Build history of the part. All positions in model axes, mm. A direction names the side the tool comes from. Round coordinates to 2 decimals unless told otherwise and drop trailing zeros. Write each loop counter-clockwise with the first axis right and the second up, starting at its lowest first coordinate (ties: lowest second). Pieces come first, ordered by that corner, then holes.
from build123d import *

# Parameters (mm, degrees)
SKETCH1_W                = 39
SKETCH1_H                = 70
BASE_DEPTH               = 4.5
SKETCH2_W                = 4
SKETCH2_H                = 62
WALLS_DEPTH              = 7.5
SKETCH3_W                = 10
SKETCH3_H                = 7.5
PWR_CONNECTOR_HOLE_DEPTH = 4
SKETCH4_W                = 7.5
SKETCH4_H                = 8
GPS_CONNECTOR_HOLE_DEPTH = 4
SKETCH5_R                = 1.25
MOUNTING_HOLES_DEPTH     = 4
GPS_MOUNT_DEPTH          = 4
SKETCH11_W               = 17
SKETCH11_H               = 1
SKETCH11_W_2             = 12
SKETCH11_H_2             = 3
PWR_CABLE_HOLDER1_DEPTH  = 4
PWR_FILLET2_R            = 1
PWR_FILLET3_R            = 0.5
SKETCH15_R               = 6
BALLON_MOUNT_DEPTH       = 70
SKETCH16_R               = 2.25
BALLOON_MOUNT_HOLE_DEPTH = 70
SKETCH21_R               = 2.25
SAFETY_MOUNT_DEPTH       = 4.5
SKETCH22_W               = 35
SKETCH22_H               = 66
LID_HOLE_DEPTH           = 7.5
SKETCH25_W               = 3.5
SKETCH25_H               = 66
CORRECTION_DEPTH         = 2
FILLET4_R                = 0.75
FILLET5_R                = 1
SKETCH12_W               = 7
SKETCH12_H               = 2.5
SKETCH12_W_2             = 2
SKETCH12_H_2             = 2
CUT_EXTRUDE2_DEPTH       = 1.99
SKETCH13_W               = 2.326586719
SKETCH13_H               = 10
CUT_EXTRUDE3_DEPTH       = 2
FILLET6_R                = 1
FILLET7_R                = 1
FILLET8_START            = 4
FILLET8_DEPTH            = 12.5
FILLET8_START_2          = 9.5
FILLET8_2_DEPTH          = 7


with BuildPart() as part:
    # Sketch1 → Base (new body)
    with BuildSketch(Plane.XY):
        with Locations((19.5, 35)):
            Rectangle(SKETCH1_W, SKETCH1_H)
    extrude(amount=BASE_DEPTH)

    # Sketch2 → Walls (add)
    with BuildSketch(Plane.XY.offset(4.5)):
        Polygon((39, 66), (39, 70), (0, 70), (0, 66), (4, 66), (35, 66), align=None)
        with Locations((37, 35)):
            Rectangle(SKETCH2_W, SKETCH2_H)
        Polygon((4, 66), (0, 66), (0, 0), (4, 0), (4, 4), align=None)
        Polygon((39, 0), (39, 4), (35, 4), (4, 4), (4, 0), align=None)
    extrude(amount=WALLS_DEPTH)

    # Sketch3 → PWR connector hole (cut)
    with BuildSketch(Plane(origin=(0, 4, 0), x_dir=(1, 0, 0), z_dir=(0, 1, 0))):
        with Locations((14.5, -8.25)):
            Rectangle(SKETCH3_W, SKETCH3_H)
    extrude(amount=-PWR_CONNECTOR_HOLE_DEPTH, mode=Mode.SUBTRACT)

    # Sketch4 → GPS connector hole (cut)
    with BuildSketch(Plane.ZY.offset(-35)):
        with Locations((8.25, 18.5)):
            Rectangle(SKETCH4_W, SKETCH4_H)
    extrude(amount=-GPS_CONNECTOR_HOLE_DEPTH, mode=Mode.SUBTRACT)

    # Sketch5 → Mounting holes (cut)
    with BuildSketch(Plane.XY.offset(4.5)):
        with Locations((7.25, 7.25)):
            Circle(SKETCH5_R)
        with Locations(Location((31.75, 7.25, 0), (0, 0, 180))):
            Circle(SKETCH5_R)
        with Locations(Location((7.25, 62.75, 0), (0, 0, 180))):
            Circle(SKETCH5_R)
    extrude(amount=-MOUNTING_HOLES_DEPTH, mode=Mode.SUBTRACT)

    # Sketch7 → GPS mount (add)
    with BuildSketch(Plane(origin=(0, 0, 0), x_dir=(-1, 0, 0), z_dir=(0, 0, -1))):
        Polygon((-39, 1), (-39, 0), (-7, 0), (-7, 18.5), (-39, 18.5), (-39, 17.5), (-8, 17.5), (-8, 1), align=None)
    extrude(amount=GPS_MOUNT_DEPTH)

    # Sketch11 → PWR cable holder1 (add)
    with BuildSketch(Plane(origin=(0, 0, 0), x_dir=(-1, 0, 0), z_dir=(0, 0, -1))):
        Polygon((-5, 0), (-3, 0), (-3, 21.5), (-5, 21.5), (-5, 20.5), align=None)
        with Locations((-13.5, 21)):
            Rectangle(SKETCH11_W, SKETCH11_H)
        with Locations((-33, 20)):
            Rectangle(SKETCH11_W_2, SKETCH11_H_2)
    extrude(amount=PWR_CABLE_HOLDER1_DEPTH)

    # PWR fillet2
    pwr_fillet2_edges = [part.edges().sort_by_distance(p)[0] for p in [
        (27, 21.5, -2),
    ]]
    fillet(pwr_fillet2_edges, radius=PWR_FILLET2_R)

    # PWR fillet3
    pwr_fillet3_edges = [part.edges().sort_by_distance(p)[0] for p in [
        (22, 21.5, -2),
        (22, 20.5, -2),
    ]]
    fillet(pwr_fillet3_edges, radius=PWR_FILLET3_R - 0.0001)  # a hair under: the kernel refuses the full size

    # Sketch15 → Ballon mount (add)
    with BuildSketch(Plane.XZ):
        with Locations((0, 6)):
            Circle(SKETCH15_R)
    extrude(amount=-BALLON_MOUNT_DEPTH)

    # Sketch16 → Balloon mount hole (cut)
    with BuildSketch(Plane.XZ):
        with Locations(Location((0, 6, 0), (0, 0, 270))):
            Circle(SKETCH16_R)
    extrude(amount=-BALLOON_MOUNT_HOLE_DEPTH, mode=Mode.SUBTRACT)

    # Sketch21 → Safety mount (cut)
    with BuildSketch(Plane.ZY.offset(6)):
        with Locations((6, 3.5)):
            Circle(SKETCH21_R)
        with Locations((6, 66.5)):
            Circle(SKETCH21_R)
    extrude(amount=-SAFETY_MOUNT_DEPTH, mode=Mode.SUBTRACT)

    # Sketch22 → Lid hole (cut)
    with BuildSketch(Plane.XY.offset(12)):
        with Locations((19.5, 35)):
            Rectangle(SKETCH22_W, SKETCH22_H)
    extrude(amount=-LID_HOLE_DEPTH, mode=Mode.SUBTRACT)

    # Sketch25 → Correction (add)
    with BuildSketch(Plane(origin=(2, 0, 0), x_dir=(0, 0, -1), z_dir=(1, 0, 0))):
        with Locations((-6.25, 35)):
            Rectangle(SKETCH25_W, SKETCH25_H)
    extrude(amount=CORRECTION_DEPTH)

    # Fillet4
    fillet4_edges = [part.edges().sort_by_distance(p)[0] for p in [
        (7, 18.5, -2),
    ]]
    fillet(fillet4_edges, radius=FILLET4_R)

    # Fillet5
    fillet5_edges = [part.edges().sort_by_distance(p)[0] for p in [
        (5, 20.5, -2),
    ]]
    fillet(fillet5_edges, radius=FILLET5_R)

    # Sketch12 → Cut-Extrude2 (cut)
    with BuildSketch(Plane.XZ):
        with Locations((13, 3.25)):
            Rectangle(SKETCH12_W, SKETCH12_H)
        Polygon((5, 4.5), (5, 2), (7, 2), (9.5, 2), (9.5, 4.5), align=None)
        with Locations((6, 1)):
            Rectangle(SKETCH12_W_2, SKETCH12_H_2)
    extrude(amount=-CUT_EXTRUDE2_DEPTH, mode=Mode.SUBTRACT)

    # Sketch13 → Cut-Extrude3 (cut)
    with BuildSketch(Plane(origin=(39, 0, 0), x_dir=(0, 0, -1), z_dir=(1, 0, 0))):
        Polygon((-2.326586719, 20.5), (-4.5, 20.5), (-4.5, 16.5), (-3.326586719, 16.5), (-2.326586719, 16.5), (-2.326586719, 17.5), align=None)
        Polygon((0, 17.5), (-2.326586719, 20.5), (-2.326586719, 17.5), align=None)
        Polygon((0, 17.5), (-2.326586719, 17.5), (-2.326586719, 16.5), (-2.326586719, 11), (0, 11), align=None)
        Polygon((-2.326586719, 16.5), (-3.326586719, 16.5), (-3.326586719, 1), (-2.326586719, 1), (-2.326586719, 11), align=None)
        with Locations((-1.16329336, 6)):
            Rectangle(SKETCH13_W, SKETCH13_H)
    extrude(amount=-CUT_EXTRUDE3_DEPTH, mode=Mode.SUBTRACT)

    # Fillet6
    fillet6_edges = [part.edges().sort_by_distance(p)[0] for p in [
        (37, 18.5, 4.5),
    ]]
    fillet(fillet6_edges, radius=FILLET6_R)

    # Fillet7
    fillet7_edges = [part.edges().sort_by_distance(p)[0] for p in [
        (6, 1.99, 0),
    ]]
    fillet(fillet7_edges, radius=FILLET7_R)

    # Fillet8: read off the stored shape, not the designer's step
    # Fillet8 outline → Fillet8 (cut)
    with BuildSketch(Plane.YZ.offset(FILLET8_START)):
        with BuildLine():
            Line((2.99, 4.5), (2, 4.5))
            Line((2, 4.5), (2, 3.64106736))
            ThreePointArc((2, 3.64106736), (2.334663201, 4.255336799), (2.99, 4.5))
        make_face()
    extrude(amount=FILLET8_DEPTH, mode=Mode.SUBTRACT)

    # Fillet8 2 outline → Fillet8 2 (cut)
    with BuildSketch(Plane.YZ.offset(FILLET8_START_2)):
        with BuildLine():
            Line((2, 3.64106736), (2, 4.5))
            Line((2, 4.5), (1.99, 4.5))
            Line((1.99, 4.5), (1.99, 3.5))
            ThreePointArc((1.99, 3.5), (1.992503133, 3.570710678), (2, 3.64106736))
        make_face()
    extrude(amount=FILLET8_2_DEPTH, mode=Mode.SUBTRACT)


solid = part.part
1) Which spindle directions (+Z, -Z, +X, -X, +Y, -Y) get a long thin tool onto all of the face, cutting with end or side? Do faces 3 (the flat face through (7, 63, 0.5)), 4 (the flat face through (14, 20.5, -2)), 5 (the flat face through (38.01, 18.98, 1.15)), 6 (the flat face through (38, 9, 3.327)), 7 (the flat face through (7, 1, 4.5)). Say none if no direction does.
Results:
face 3: +Z
face 4: -Z
face 5: +Z, +X
face 6: -Z, +X
face 7: -Y
2) Slice it at C-C (x = 31.75). Write the cut outline in (y, z).
Results:
outline: (0, -4) - (1, -4) - (1, 0) - (17.5, 0) - (17.5, -4) - (21.5, -4) - (21.5, 0) - (70, 0) - (70, 12) - (68, 12) - (68, 4.5) - (8.5, 4.5) - (8.5, 0.5) - (6, 0.5) - (6, 4.5) - (2, 4.5) - (2, 12) - (0, 12) - close
3) Wall check: L1, parallel to Y at x = -3.25, z = 6; L2, parallel to Y at x = 7.25, z = 2.75; L3, parallel to X at y = 20.5, z = 6. Give the ranges that are in metal, low to high.
Results:
L1: y = 0 to 1.25, 5.75 to 64.25, 68.75 to 70
L2: y = 1.99 to 6, 8.5 to 61.5, 64 to 70
L3: x = -6 to -2.25, 2 to 4
4) Slice it at A-A (z = 6). Count the separate pieces of the cut face and the enclosed holes in it, plus the area to 3 significant figures.
Results:
separate pieces: 5
enclosed holes: 0
area: 604 mm2
5) Mould opens along Y. For faces 1 (the flat face through (22, 9, 0)), 2 (the flat face through (27, 19, -2)) say: released by +Y, released by -Y, zero draft, split by the parting line, or undercut.
Results:
face 1: undercut
face 2: zero draft
6) Pin check, flat tips, straight feed: pin 1 Ø0.8 at (x, y) = (7, 7) entering from +Z; pin 2 Ø4 at (x, y) = (17.5, 58) entering from +Z; pin 3 Ø0.6 at (y, z) = (3, 8) entering from -X; pin 4 Ø4 at (y, z) = (40.5, 7) entering from -X. Stop position of each tip, or through.
Results:
pin 1: stops at z = 0.5
pin 2: stops at z = 4.5
pin 3: stops at x = -5.62
pin 4: stops at x = -6
